```python
from build123d import *

# Parameters (mm, degrees)
SZKIC1_W                        = 42.6
SZKIC1_H                        = 25
DODANIE_WYCI_GNI_CIE2_DEPTH     = 18
SKORUPA5_T                      = -2
SZKIC2_R                        = 1.3
DODANIE_WYCI_GNI_CIE3_DEPTH     = 2
SZKIC3_R                        = 4.9
SZKIC3_R_2                      = 2.5
WYTNIJ_WYCI_GNI_CIE1_DEPTH      = 2
WYTNIJ_WYCI_GNI_CIE2_DEPTH      = 53.402385442
WYTNIJ_WYCI_GNI_CIE2_DEPTH_BACK = 53.402385442
SZKIC4_W                        = 15
SZKIC4_H                        = 13


with BuildPart() as part:
    # Szkic1 → Dodanie-wyciągnięcie2 (new body)
    with BuildSketch(Plane(origin=(0, 0, 0), x_dir=(1, 0, 0), z_dir=(0, 1, 0))):
        Rectangle(SZKIC1_W, SZKIC1_H)
    extrude(amount=DODANIE_WYCI_GNI_CIE2_DEPTH)

    # Skorupa5
    skorupa5_openings = [part.faces().sort_by_distance(p)[0] for p in [
        (0, 18, 0),
        (0, 9, -12.5),
        (0, 9, 12.5),
    ]]
    offset(amount=SKORUPA5_T, openings=skorupa5_openings, kind=Kind.INTERSECTION)

    # Szkic2 → Dodanie-wyciągnięcie3 (add)
    # profile 1 of 4: a face of its own
    with BuildSketch(Plane(origin=(0, 18, 0), x_dir=(1, 0, 0), z_dir=(0, 1, 0))):
        with BuildLine():
            Line((-21.3, 12.5), (-24.3, 12.5))
            ThreePointArc((-24.3, 12.5), (-25.714213562, 11.914213562), (-26.3, 10.5))
            Line((-26.3, 10.5), (-26.3, 9.5))
            ThreePointArc((-26.3, 9.5), (-25.714213562, 8.085786438), (-24.3, 7.5))
            Line((-24.3, 7.5), (-21.3, 7.5))
            Line((-21.3, 7.5), (-21.3, 12.5))
        make_face()
        with Locations(Location((-23.8, 10, 0), (0, 0, 270))):
            Circle(SZKIC2_R, mode=Mode.SUBTRACT)
    # profile 2 of 4: a face of its own
    with BuildSketch(Plane(origin=(0, 18, 0), x_dir=(1, 0, 0), z_dir=(0, 1, 0))):
        with BuildLine():
            Line((-21.3, -7.5), (-24.3, -7.5))
            ThreePointArc((-24.3, -7.5), (-25.714213562, -8.085786438), (-26.3, -9.5))
            Line((-26.3, -9.5), (-26.3, -10.5))
            ThreePointArc((-26.3, -10.5), (-25.714213562, -11.914213562), (-24.3, -12.5))
            Line((-24.3, -12.5), (-21.3, -12.5))
            Line((-21.3, -12.5), (-21.3, -7.5))
        make_face()
        with Locations(Location((-23.8, -10, 0), (0, 0, 90))):
            Circle(SZKIC2_R, mode=Mode.SUBTRACT)
    # profile 3 of 4: a face of its own
    with BuildSketch(Plane(origin=(0, 18, 0), x_dir=(1, 0, 0), z_dir=(0, 1, 0))):
        with BuildLine():
            Line((21.3, -12.5), (21.3, -7.5))
            Line((21.3, -7.5), (24.3, -7.5))
            ThreePointArc((24.3, -7.5), (25.714213562, -8.085786438), (26.3, -9.5))
            Line((26.3, -9.5), (26.3, -10.5))
            ThreePointArc((26.3, -10.5), (25.714213562, -11.914213562), (24.3, -12.5))
            Line((24.3, -12.5), (21.3, -12.5))
        make_face()
        with Locations(Location((23.8, -10, 0), (0, 0, 270))):
            Circle(SZKIC2_R, mode=Mode.SUBTRACT)
    # profile 4 of 4: a face of its own
    with BuildSketch(Plane(origin=(0, 18, 0), x_dir=(1, 0, 0), z_dir=(0, 1, 0))):
        with BuildLine():
            Line((21.3, 7.5), (24.3, 7.5))
            ThreePointArc((24.3, 7.5), (25.714213562, 8.085786438), (26.3, 9.5))
            Line((26.3, 9.5), (26.3, 10.5))
            ThreePointArc((26.3, 10.5), (25.714213562, 11.914213562), (24.3, 12.5))
            Line((24.3, 12.5), (21.3, 12.5))
            Line((21.3, 12.5), (21.3, 7.5))
        make_face()
        with Locations(Location((23.8, 10, 0), (0, 0, 90))):
            Circle(SZKIC2_R, mode=Mode.SUBTRACT)
    extrude(amount=-DODANIE_WYCI_GNI_CIE3_DEPTH)

    # Szkic3 → Wytnij-wyciągnięcie1 (cut)
    with BuildSketch(Plane(origin=(0, 2, 0), x_dir=(1, 0, 0), z_dir=(0, 1, 0))):
        with Locations(Location((-12.3, 0, 0), (0, 0, 270))):
            Circle(SZKIC3_R)
        with Locations(Location((12.3, 0, 0), (0, 0, 270))):
            Circle(SZKIC3_R)
        with Locations(Location((0, 7, 0), (0, 0, 270))):
            Circle(SZKIC3_R_2)
        with Locations(Location((0, -7, 0), (0, 0, 270))):
            Circle(SZKIC3_R_2)
    extrude(amount=-WYTNIJ_WYCI_GNI_CIE1_DEPTH, mode=Mode.SUBTRACT)

    # Szkic4 → Wytnij-wyciągnięcie2 (cut, two sides: drawn at the far end of the back side and taken through both)
    with BuildSketch(Plane.ZY.offset(21.3).offset(-WYTNIJ_WYCI_GNI_CIE2_DEPTH_BACK)):
        with Locations((0, 11.5)):
            Rectangle(SZKIC4_W, SZKIC4_H)
    extrude(amount=WYTNIJ_WYCI_GNI_CIE2_DEPTH + WYTNIJ_WYCI_GNI_CIE2_DEPTH_BACK, mode=Mode.SUBTRACT)


solid = part.part
```
Can you work these out from the model? Positions are in its coordinate system, mm. A direction names the side the tool comes from. Round coordinates to 2 decimals unless told otherwise and drop trailing zeros. Loops run counter-clockwise (first coordinate to the right, second up) from the corner with the lowest first, then second, coordinate; pieces in that order, holes last. Notation, with made-up numbers: (41.5, 39.5) -> (61.5, 39.5) arc R10 cw to (61.5, 48.5) -> close; hole circle Ø2 at (-30, 80.5). An arc over 180 degrees is marked (long way). One line per item, written item: value. Start each with the question number.
1. If we section it at B-B, the plane x = 0: Write out the boundary of the cut face in (y, z), then the cut area to 3 significant figures.
2. If we mould it in two halves opening along Z, with no side actions, what happens to faces 5 (the flat face through (21, 11, -7.5)), 6 (the flat face through (-26.3, 17, 10)), 7 (the cylindrical face through (-25.7, 17.01, -11.93)), 8 (the cylindrical face through (-25.73, 17.01, 11.9))? For each: pulls with the +Z half, pulls with the -Z half, needs draft (parallel to the pull), parting line crosses it, or undercut.
3. If I drill on probe 1 along X at (y, z) = (17.3, 10); probe 2 along X at (y, z) = (1.3, -7); probe 3 along X at (y, z) = (4, -10.25), over which ranges is the centre line in solid material (lowest first)?
4. For pin 1 (11.5 mm diameter, centred on x = -12.3, z = 0, fed in from +Y); pin 2 (1 mm diameter, centred on y = 2.5, z = 2.5, fed in from -X); pin 3 (3.5 mm diameter, centred on x = 23.8, z = 10, fed in from -Y), each with a flat end and sliding along its axis, tell me the tip position at first contact or that it passes through.
5. If we section it at D-D, the plane x = -23.8: Write out the boundary of the cut face in (y, z).
6. If we section it at A-A, the plane z = -7: Write out the boundary of the cut face in (x, y).
7. For faces 1 (the flat face through (22.7, 16, 8.9)), 2 (the flat face through (-19.3, 4.6, 0.2)), 3 (the cylindrical face through (-25.73, 17.01, -8.1)), 4 (the cylindrical face through (25.7, 17.01, 8.07)), which set-ups out of +Z, -Z, +X, -X, +Y, -Y let a thin tool reach every point of the face, with its end or its side?
8. If we section it at C-C, the plane y = 6.75: Write out the boundary of the cut face in (x, z), then the cut area to 3 significant figures.
Calculated:
1. outline: (0, -12.5) -> (2, -12.5) -> (2, -9.5) -> (0, -9.5) -> close; (0, -4.5) -> (2, -4.5) -> (2, 4.5) -> (0, 4.5) -> close; (0, 9.5) -> (2, 9.5) -> (2, 12.5) -> (0, 12.5) -> close
1. area: 30.0 mm²
2. face 5: undercut
2. face 6: needs draft
2. face 7: pulls with the -Z half
2. face 8: pulls with the +Z half
3. probe 1: x = -26.3 to -25.1, -22.5 to -19.3, 19.3 to 22.5, 25.1 to 26.3
3. probe 2: x = -21.3 to -2.5, 2.5 to 21.3
3. probe 3: x = -21.3 to -19.3, 19.3 to 21.3
4. pin 1: stops at y = 2
4. pin 2: stops at x = -21.3
4. pin 3: stops at y = 16
5. outline: (16, -12.5) -> (18, -12.5) -> (18, -11.3) -> (16, -11.3) -> close; (16, -8.7) -> (18, -8.7) -> (18, -7.5) -> (16, -7.5) -> close; (16, 7.5) -> (18, 7.5) -> (18, 8.7) -> (16, 8.7) -> close; (16, 11.3) -> (18, 11.3) -> (18, 12.5) -> (16, 12.5) -> close
6. outline: (-21.3, 0) -> (-2.5, 0) -> (-2.5, 2) -> (-19.3, 2) -> (-19.3, 5) -> (-21.3, 5) -> close; (2.5, 0) -> (21.3, 0) -> (21.3, 5) -> (19.3, 5) -> (19.3, 2) -> (2.5, 2) -> close
7. face 1: +Z, -Z, +X, -Y
7. face 2: +Z, -Z, +Y
7. face 3: -X, +Y, -Y
7. face 4: +X, +Y, -Y
8. outline: (-21.3, -12.5) -> (-19.3, -12.5) -> (-19.3, -7.5) -> (-21.3, -7.5) -> close; (-21.3, 7.5) -> (-19.3, 7.5) -> (-19.3, 12.5) -> (-21.3, 12.5) -> close; (19.3, -12.5) -> (21.3, -12.5) -> (21.3, -7.5) -> (19.3, -7.5) -> close; (19.3, 7.5) -> (21.3, 7.5) -> (21.3, 12.5) -> (19.3, 12.5) -> close
8. area: 40.0 mm²
